The model under review builds one solid part; all positions refer to its coordinate system, in mm. A direction names the side the tool comes from. Coordinates: 2 decimals unless noted, no trailing zeros. Order: outer loops, then holes, each group sorted by start corner. A loop starts at its lowest first (then second) coordinate and runs counter-clockwise, first axis right, second up. Notation, with made-up numbers: M 57.5,38 L 96.5,38 A18 ccw 96.5,68 Z; hole C -37,33 d11. An arc over 180 degrees is marked long. One line per item, written item: value.
```python
from build123d import *

# Parameters (mm, degrees)
SKETCH018_AS_DRAWN_R                 = 3.15
EXTRUDE021_DEPTH                     = 5
EXTRUDE021_ONTO_SKETCH018_ROLL_ANGLE = 90
SKETCH007_AS_DRAWN_R                 = 1.8
EXTRUDE020_DEPTH                     = 15
EXTRUDE020_ONTO_SKETCH007_ROLL_ANGLE = 90
SKETCH005_AS_DRAWN_R                 = 1.8
SKETCH005_AS_DRAWN_R_2               = 1.3
EXTRUDE008_DEPTH                     = 40
EXTRUDE008_ONTO_SKETCH005_ROLL_ANGLE = 90
SKETCH006_AS_DRAWN_R                 = 3.25
EXTRUDE009_DEPTH                     = 4
EXTRUDE009_ONTO_SKETCH006_ROLL_ANGLE = 90
SKETCH019_AS_DRAWN_R                 = 3.25
EXTRUDE022_DEPTH                     = 10
EXTRUDE022_ONTO_SKETCH019_ROLL_ANGLE = 90
SKETCH004_R                          = 12.5
EXTRUDE007_DEPTH                     = 60
EXTRUDE001_DEPTH                     = 10
EXTRUDE_DEPTH                        = 45
CHAMFER_SIZE                         = 0.7


with BuildPart() as extrude021:
    # Sketch018 as drawn → Extrude021 (new)
    with BuildSketch(Plane.XY):
        with Locations((0, 20)):
            Circle(SKETCH018_AS_DRAWN_R)
    extrude(amount=-EXTRUDE021_DEPTH)


with BuildPart() as extrude021_1:
    # Extrude021 onto Sketch018 roll: moved
    add(extrude021.part.rotate(Axis((0, 0, 0), (1, 0, 0)), EXTRUDE021_ONTO_SKETCH018_ROLL_ANGLE))


with BuildPart() as extrude021_2:
    # Extrude021 onto Sketch018 placement: moved
    add(extrude021_1.part.moved(Location((0, -55, 0))))


with BuildPart() as bottomscrewhole:
    # Sketch007 as drawn → Extrude020 (new)
    with BuildSketch(Plane.XY):
        with Locations((0, 20)):
            Circle(SKETCH007_AS_DRAWN_R)
    extrude(amount=-EXTRUDE020_DEPTH)


with BuildPart() as bottomscrewhole_1:
    # Extrude020 onto Sketch007 roll: moved
    add(bottomscrewhole.part.rotate(Axis((0, 0, 0), (1, 0, 0)), EXTRUDE020_ONTO_SKETCH007_ROLL_ANGLE))


with BuildPart() as bottomscrewhole_2:
    # Extrude020 onto Sketch007 placement: moved
    add(bottomscrewhole_1.part.moved(Location((0, -55, 0))))

    # Fusion006: union Extrude021
    add(extrude021_2.part)


with BuildPart() as extrude008:
    # Sketch005 as drawn → Extrude008 (new)
    with BuildSketch(Plane.XY):
        with Locations((-16, 10)):
            Circle(SKETCH005_AS_DRAWN_R)
        with Locations((16, 10)):
            Circle(SKETCH005_AS_DRAWN_R)
        with Locations((16, -10)):
            Circle(SKETCH005_AS_DRAWN_R)
        with Locations((-16, -10)):
            Circle(SKETCH005_AS_DRAWN_R)
        with Locations((0, 17.5)):
            Circle(SKETCH005_AS_DRAWN_R_2)
    extrude(amount=-EXTRUDE008_DEPTH)


with BuildPart() as extrude008_1:
    # Extrude008 onto Sketch005 roll: moved
    add(extrude008.part.rotate(Axis((0, 0, 0), (1, 0, 0)), EXTRUDE008_ONTO_SKETCH005_ROLL_ANGLE))


with BuildPart() as extrude008_2:
    # Extrude008 onto Sketch005 placement: moved
    add(extrude008_1.part)


with BuildPart() as extrude008_3:
    # Extrude008 placement: moved
    add(extrude008_2.part.moved(Location((0, -20, 0))))


with BuildPart() as extrude009:
    # Sketch006 as drawn → Extrude009 (new)
    with BuildSketch(Plane.XY):
        with Locations((-16, 10)):
            Circle(SKETCH006_AS_DRAWN_R)
        with Locations((16, 10)):
            Circle(SKETCH006_AS_DRAWN_R)
        with Locations((16, -10)):
            Circle(SKETCH006_AS_DRAWN_R)
        with Locations((-16, -10)):
            Circle(SKETCH006_AS_DRAWN_R)
    extrude(amount=EXTRUDE009_DEPTH)


with BuildPart() as extrude009_1:
    # Extrude009 onto Sketch006 roll: moved
    add(extrude009.part.rotate(Axis((0, 0, 0), (1, 0, 0)), EXTRUDE009_ONTO_SKETCH006_ROLL_ANGLE))


with BuildPart() as extrude009_2:
    # Extrude009 onto Sketch006 placement: moved
    add(extrude009_1.part)


with BuildPart() as extrude009_3:
    # Extrude009 placement: moved
    add(extrude009_2.part.moved(Location((0, 8, 0))))


with BuildPart() as screwholes:
    # Sketch019 as drawn → Extrude022 (new)
    with BuildSketch(Plane.XY):
        with Locations((0, 17.5)):
            Circle(SKETCH019_AS_DRAWN_R)
    extrude(amount=-EXTRUDE022_DEPTH)


with BuildPart() as screwholes_1:
    # Extrude022 onto Sketch019 roll: moved
    add(screwholes.part.rotate(Axis((0, 0, 0), (1, 0, 0)), EXTRUDE022_ONTO_SKETCH019_ROLL_ANGLE))


with BuildPart() as screwholes_2:
    # Extrude022 onto Sketch019 placement: moved
    add(screwholes_1.part)


with BuildPart() as screwholes_3:
    # Extrude022 placement: moved
    add(screwholes_2.part.moved(Location((0, -8, 0))))

    # Fusion007: union Extrude008, Extrude009
    add(extrude008_3.part)
    add(extrude009_3.part)


with BuildPart() as screwholes_4:
    # Fusion007 placement: moved
    add(screwholes_3.part.moved(Location((0, 0, 22.5))))


with BuildPart() as tube:
    # Sketch004 → Extrude007 (new body)
    with BuildSketch(Plane(origin=(0, 16, 0), x_dir=(1, 0, 0), z_dir=(0, 0, 1))):
        Circle(SKETCH004_R)
    extrude(amount=EXTRUDE007_DEPTH)


with BuildPart() as tube_1:
    # Extrude007 placement: moved
    add(tube.part.moved(Location((0, 0, -12.5))))


with BuildPart() as extrude001:
    # Sketch → Extrude001 (new body)
    with BuildSketch(Plane.YZ):
        Polygon((0, 40), (0, 0), (-55, 0), (-55, 25), (-45, 25), (-45, 14.75), (-20, 14.75), align=None)
    extrude(amount=EXTRUDE001_DEPTH)


with BuildPart() as extrude001_1:
    # Extrude001 placement: moved
    add(extrude001.part.moved(Location((-5, 0, 0))))


with BuildPart() as chamfer_body:
    # Sketch003 → Extrude (new body)
    with BuildSketch(Plane.XY):
        Polygon((21, 14.910553), (21, 5), (14, 5), (5, 0), (-5, 0), (-14, 5), (-21, 5), (-21, 16), (-12.5, 16), (-11.410553, 14.910553), (12.452434, 14.910553), align=None)
    extrude(amount=EXTRUDE_DEPTH)

    # Fusion: union Extrude001
    add(extrude001_1.part)

    # Cut: cut tube
    add(tube_1.part, mode=Mode.SUBTRACT)

    # Cut001: cut ScrewHoles
    add(screwholes_4.part, mode=Mode.SUBTRACT)

    # Cut002: cut BottomScrewHole
    add(bottomscrewhole_2.part, mode=Mode.SUBTRACT)

    # Chamfer
    chamfer_edges = [chamfer_body.edges().sort_by_distance(p)[0] for p in [
        (12.452434, 14.910553, 22.5),
        (16.726217, 14.910553, 0),
        (16.726217, 14.910553, 45),
        (21, 14.910553, 22.5),
        (-0.545242, 3.511897, 0),
        (-0.545242, 3.511897, 45),
        (-12.5, 16, 22.5),
        (-16.75, 16, 0),
        (-16.75, 16, 45),
        (-21, 16, 22.5),
    ]]
    chamfer(chamfer_edges, length=CHAMFER_SIZE)


solid = chamfer_body.part
```
(1) Insertion check: pin 1 Ø4 at (x, z) = (-16, 32.5) entering from -Y; pin 2 Ø3 at (x, z) = (-0.5, 41) entering from -Y; pin 3 Ø8.5 at (x, z) = (-16, 12.5) entering from -Y. Each pin has a flat end and moves straight along its axis. Give the tip position at first contact, or say it passes through.
Geometry results:
pin 1: stops at y = 8
pin 2: stops at y = 2
pin 3: stops at y = 3.75
(2) For L1, parallel to Z at x = -16, y = 14; L2, parallel to Z at x = 16, y = 5.6; L3, parallel to X at y = 6, z = 12, list the stretches that pass through material, from the lowest coordinate up.
Geometry results:
L1: z = 0 to 10.7, 14.3 to 30.7, 34.3 to 45
L2: z = 0 to 9.25, 15.75 to 29.25, 35.75 to 45
L3: x = -21 to -19.21, -12.79 to -7.5, 7.5 to 12.79, 19.21 to 21
(3) We need section D-D, the plane x = -16. State the section outline as (y, z) points, plus the area to 3 significant figures.
Geometry results:
outline: M 5,0 L 15.3,0 L 16,0.7 L 16,10.7 L 8,10.7 L 8,9.25 L 5,9.25 Z; M 5,15.75 L 8,15.75 L 8,14.3 L 16,14.3 L 16,30.7 L 8,30.7 L 8,29.25 L 5,29.25 Z; M 5,35.75 L 8,35.75 L 8,34.3 L 16,34.3 L 16,44.3 L 15.3,45 L 5,45 Z
area: 398 mm2
(4) We need section A-A, the plane x = 16. State the section outline as (y, z) points.
Geometry results:
outline: M 5,0 L 14.21,0 L 14.91,0.7 L 14.91,10.7 L 8,10.7 L 8,9.25 L 5,9.25 Z; M 5,15.75 L 8,15.75 L 8,14.3 L 14.91,14.3 L 14.91,30.7 L 8,30.7 L 8,29.25 L 5,29.25 Z; M 5,35.75 L 8,35.75 L 8,34.3 L 14.91,34.3 L 14.91,44.3 L 14.21,45 L 5,45 Z
(5) Tool access review of faces 4 (the flat face through (0, 0, 44)), 5 (the flat face through (-5, -27, 11)), 6 (the flat face through (-2, -45, 20)), 7 (the cylindrical face through (-0.234, -47.535, 21.785)), 8 (the flat face through (-4, 3, 45)): name each direction out of +Z, -Z, +X, -X, +Y, -Y from which nothing blocks a thin tool from reaching the whole face with its end or side.
Geometry results:
face 4: +Z, +X, -X, -Y
face 5: +Z, -Z, -X, -Y
face 6: +Z, +X, -X
face 7: -Y
face 8: +Z, +X, -X, +Y, -Y
(6) Mouldability with a two-part tool opening along Y and no side actions: class faces 1 (the flat face through (0, -33, 14.75)), 2 (the flat face through (-17, 16, 22)), 3 (the flat face through (5, -27, 11)) as +Y half, -Y half, draft (parallel to the pull), parting line (faces both ways), or undercut.
Geometry results:
face 1: undercut
face 2: +Y half
face 3: draft
(7) We need section B-B, the plane z = 12.5. Count the separate pieces of the cut face and the enclosed holes in it, plus the area to 3 significant figures.
Geometry results:
separate pieces: 3
enclosed holes: 0
area: 758 mm2
(8) We need section C-C, the plane z = 6.5. State the section outline as (x, y) points, plus the area to 3 significant figures.
Geometry results:
outline: M -21,5 L -14,5 L -5,0 L -5,-55 L 5,-55 L 5,0 L 14,5 L 21,5 L 21,14.21 L 20.3,14.91 L 13.15,14.91 L 12.37,14.22 A12.5 cw -12.48,15.3 L -13.2,16 L -20.3,16 L -21,15.3 Z
area: 851 mm2
